```python
from build123d import *

# Parameters (mm, degrees)
SKETCH3_W         = 0.79
SKETCH3_H         = 3.1
SKETCH4_W         = 0.395
SKETCH4_H         = 0.395
CIRPATTERN1_COUNT = 2
CIRPATTERN1_ANGLE = 90


with BuildPart() as part:
    # BodySke → Base-Revolve (revolve)
    with BuildSketch(Plane.XY):
        Polygon((0, 0), (0, 2.75), (0.45, 2.75), (1.7, 1.5), (30, 1.5), (30, 0), align=None)
    revolve(axis=Axis((-6.35, 0, 0), (1, 0, 0)))

    # Sketch3 → Cross section 0
    with BuildSketch(Plane.ZY):
        Rectangle(SKETCH3_W, SKETCH3_H)
    # Sketch4 → Cross section 1
    with BuildSketch(Plane.ZY.offset(-2.08)):
        Rectangle(SKETCH4_W, SKETCH4_H)
    cross = loft(mode=Mode.SUBTRACT)

    # CirPattern1: Cross ×2 about axis
    cirpattern1_axis = Axis((0, 0, 0), (1, 0, 0))
    for i in range(1, CIRPATTERN1_COUNT):
        add(cross.rotate(cirpattern1_axis, i * CIRPATTERN1_ANGLE / (CIRPATTERN1_COUNT - 1)), mode=Mode.SUBTRACT)


solid = part.part
```
Check sheet for the modelled part. Datum: model origin and axes. Units: mm. A direction names the side the tool comes from. Coordinates: 2 decimals unless noted, no trailing zeros. Order: outer loops, then holes, each group sorted by start corner. A loop starts at its lowest first (then second) coordinate and runs counter-clockwise, first axis right, second up. Notation, with made-up numbers: (-34, 17) -> (-20, 17) arc R17 ccw to (-20, 38) -> close; hole circle Ø8 at (-16, 61). An arc over 180 degrees is marked (long way). Write item = value, one per line. Start each with the question number.
1) Material ranges on L1, parallel to Y at x = 8.5, z = 0.45; L2, parallel to Z at x = 8, y = -1.25; L3, parallel to Z at x = 26, y = -0.3, recorded low to high.
2) Cross-section at A-A (x = 15). Enter the section's corners in (y, z), then the cut area to 3 significant figures.
3) Go/stop test with flat-tipped pins: P1, Ø1, axis at x = 6, z = -1, coming from the +Y side; P2, Ø1, axis at y = 1, z = 2, coming from the +X side; P3, Ø1, axis at x = 11.5, y = 1, coming from the -Z side. Record where each tip stops, or that it passes through.
4) Access from +Z, -Z, +X, -X, +Y, -Y to the whole of each face (thin tool, end or side, straight path). Record for faces 1 (the cylindrical face through (0.228, -0.596, -2.685)), 2 (the cylindrical face through (16.05, -1.5, 0.07)).
Ans:
q1.L1 = -1.43 to 1.43
q1.L2 = -0.83 to 0.83
q1.L3 = -1.47 to 1.47
q2.outline = circle Ø3 at (0, 0)
q2.area = 7.07 mm²
q3.P1 = 1.41
q3.P2 = 1.46
q3.P3 = -1.41
q4.face_1 = +X, -X
q4.face_2 = +X
